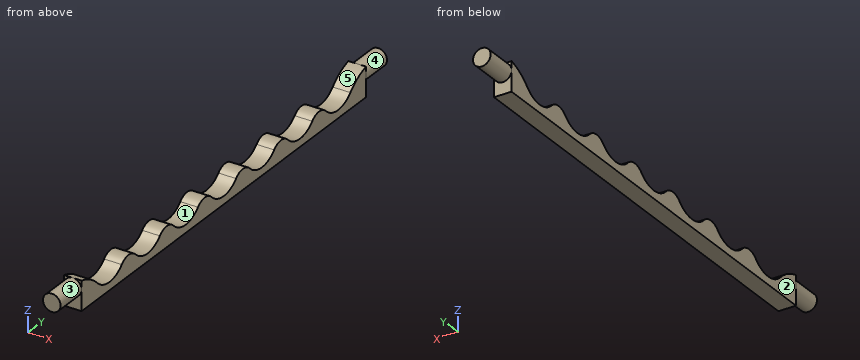
```python
from build123d import *

# Parameters (mm, degrees)
BOSS_EXTRUDE1_DEPTH = 9
SKETCH2_R           = 4.5
BOSS_EXTRUDE2_DEPTH = 16.5


with BuildPart() as part:
    # Sketch1 → Boss-Extrude1 (new body)
    with BuildSketch(Plane.YZ):
        with BuildLine():
            Line((-112, -2.5), (-112, -17.5))
            Line((-112, -17.5), (112, -17.5))
            Line((112, -17.5), (112, -2.5))
            ThreePointArc((112, -2.5), (105.325857912, -5.092638652), (99.642857143, -9.448031865))
            ThreePointArc((99.642857143, -9.448031865), (90, -13.5), (80.357142857, -9.448031865))
            ThreePointArc((80.357142857, -9.448031865), (75, -7.196938457), (69.642857143, -9.448031865))
            ThreePointArc((69.642857143, -9.448031865), (60, -13.5), (50.357142857, -9.448031865))
            ThreePointArc((50.357142857, -9.448031865), (45, -7.196938457), (39.642857143, -9.448031865))
            ThreePointArc((39.642857143, -9.448031865), (30, -13.5), (20.357142857, -9.448031865))
            ThreePointArc((20.357142857, -9.448031865), (15, -7.196938457), (9.642857143, -9.448031865))
            ThreePointArc((9.642857143, -9.448031865), (0, -13.5), (-9.642857143, -9.448031865))
            ThreePointArc((-9.642857143, -9.448031865), (-15, -7.196938457), (-20.357142857, -9.448031865))
            ThreePointArc((-20.357142857, -9.448031865), (-30, -13.5), (-39.642857143, -9.448031865))
            ThreePointArc((-39.642857143, -9.448031865), (-45, -7.196938457), (-50.357142857, -9.448031865))
            ThreePointArc((-50.357142857, -9.448031865), (-60, -13.5), (-69.642857143, -9.448031865))
            ThreePointArc((-69.642857143, -9.448031865), (-75, -7.196938457), (-80.357142857, -9.448031865))
            ThreePointArc((-80.357142857, -9.448031865), (-90, -13.5), (-99.642857143, -9.448031865))
            ThreePointArc((-99.642857143, -9.448031865), (-105.325857912, -5.092638652), (-112, -2.5))
        make_face()
    extrude(amount=BOSS_EXTRUDE1_DEPTH)

    # Sketch2 → Boss-Extrude2 (add)
    with BuildSketch(Plane.XZ.offset(112)):
        with Locations(Location((4.5, -7, 0), (0, 0, 90))):
            Circle(SKETCH2_R)
    boss_extrude2 = extrude(amount=BOSS_EXTRUDE2_DEPTH)

    # Mirror1: Boss-Extrude2 across plane
    add(boss_extrude2.mirror(Plane.ZX))


solid = part.part
```
Can you work these out from the model? Positions are in its coordinate system, mm. Face numbers are marked on the shaded views. A direction names the side the tool comes from. Round coordinates to 2 decimals unless told otherwise and drop trailing zeros. Loops run counter-clockwise (first coordinate to the right, second up) from the corner with the lowest first, then second, coordinate; pieces in that order, holes last. Notation, with made-up numbers: M 20.5,-13.5 L 30.5,-13.5 A11 ccw 30.5,-1.5 Z; hole C 53,-8 d5. An arc over 180 degrees is marked long. Write item = value, one per line. Start each with the question number.
(1) Which directions (+Z, -Z, +X, -X, +Y, -Y) give clear straight access to the entire face, cutting with the end or side of a thin tool? Please do the marked faces 3, 4 and 5.
(2) If we mould it in two halves opening along Y, with no side actions, what happens to the marked faces 1 and 2? For each: released by +Y, released by -Y, zero draft, split by the parting line, or undercut.
(3) Suppose I cut it at A-A on z = -4.75. Write out the boundary of the cut face in (x, y), plus the area to 3 significant figures.
(4) Suppose I cut it at B-B on y = 53. Write out the boundary of the cut face in (x, z).
(5) Suppose I cut it at C-C on y = 109. Write out the boundary of the cut face in (x, z).
(6) I'm going to push flat-ended pins straight in: P1, Ø2, axis at x = 7, z = -15, coming from the -Y side; P2, Ø4.5, axis at x = 5, z = -12, coming from the +Y side; P3, Ø1, axis at x = 5.5, y = -46, coming from the +Z side. Where does each tip first touch, or does it pass through?
(7) I need wall thicknesses on line 1 along Y through (x, z) = (5.5, -14.25); line 2 along Y through (x, z) = (2.5, -6.75); line 3 along Y through (x, z) = (8, -5.5). Which ranges of each line are inside material? Lowest first, please.
Answer block:
q1.face_3 = -Y
q1.face_4 = +Y
q1.face_5 = +Z, +X, -X
q2.face_1 = undercut
q2.face_2 = zero draft
q3.outline = M 0,-112 L 0.6,-112 L 0.6,-128.5 L 8.4,-128.5 L 8.4,-112 L 9,-112 L 9,-105.96 L 0,-105.96 Z; M 0,105.96 L 9,105.96 L 9,112 L 8.4,112 L 8.4,128.5 L 0.6,128.5 L 0.6,112 L 0,112 Z
q3.area = 366 mm²
q4.outline = M 0,-17.5 L 9,-17.5 L 9,-11.54 L 0,-11.54 Z
q5.outline = M 0,-17.5 L 9,-17.5 L 9,-3.4 L 0,-3.4 Z
q6.P1 = -112
q6.P2 = 128.5
q6.P3 = -7.21
q7.line_1 = -112 to 112
q7.line_2 = -128.5 to -102.75, 102.75 to 128.5
q7.line_3 = -128.5 to -104.63, 104.63 to 128.5
